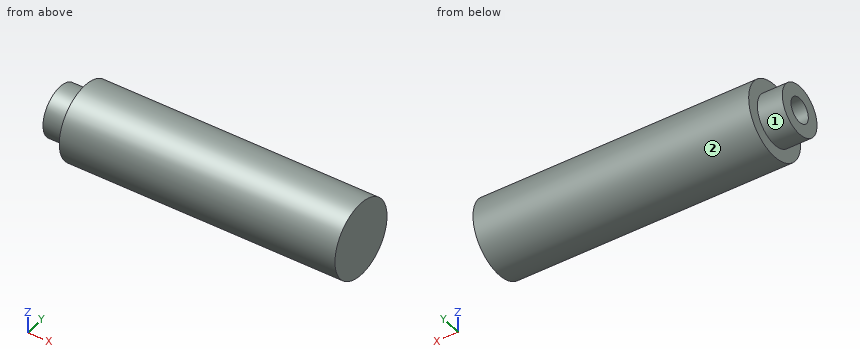
from build123d import *


with BuildPart() as part:
    # Esboço1 → Revolução1 (revolve)
    with BuildSketch(Plane.XY, mode=Mode.PRIVATE) as revolu_o1_sk:
        Polygon((-15.245, 0), (-15.245, 2.5), (-30.125, 2.5), (-30.125, 5), (-25.125, 5), (-25.125, 7.5), (30.125, 7.5), (30.125, 0), align=None)
    revolve(revolu_o1_sk.sketch.rotate(Axis((0, 0, 0), (1, 0, 0)), 90), axis=Axis((0, 0, 0), (1, 0, 0)))


solid = part.part
Could you check a few things on this model? Use its own coordinates, in mm. Face numbers are marked on the shaded views. A direction names the side the tool comes from. Coordinates: 2 decimals unless noted, no trailing zeros. Loops run counter-clockwise (first coordinate to the right, second up) from the corner with the lowest first, then second, coordinate; pieces in that order, holes last. Notation, with made-up numbers: (32.5, 12.25) -> (78.5, 12.25) arc R15 cw to (78.5, 23.25) -> close; hole circle Ø9 at (65.5, 67.5). An arc over 180 degrees is marked (long way). Answer in a Markdown table with one row per item.
(1) Imagine slicing it at A-A (y = 0). List the corners of the cut face in (x, z) for me (3 decimals), plus the area to 3 significant figures.
Results found:
| item | result |
|---|---|
| outline | (-30.125, -5) -> (-25.125, -5) -> (-25.125, -7.5) -> (30.125, -7.5) -> (30.125, 7.5) -> (-25.125, 7.5) -> (-25.125, 5) -> (-30.125, 5) -> (-30.125, 2.5) -> (-15.245, 2.5) -> (-15.245, -2.5) -> (-30.125, -2.5) -> close |
| area | 804 mm^2 |
(2) Imagine slicing it at C-C (x = -20). List the corners of the cut face in (y, z) for me, plus the area to 3 significant figures.
Results found:
| item | result |
|---|---|
| outline | circle Ø15 at (0, 0); hole circle Ø5 at (0, 0) |
| area | 157 mm^2 |
(3) If I drill on probe 1 along Z at (x, y) = (-17.5, 0.25); probe 2 along Y at (x, z) = (-18.5, 0); probe 3 along Y at (x, z) = (-26.25, 0), over which ranges is the centre line in solid material (lowest first)?
Results found:
| item | result |
|---|---|
| probe 1 | z = -7.5 to -2.49, 2.49 to 7.5 |
| probe 2 | y = -7.5 to -2.5, 2.5 to 7.5 |
| probe 3 | y = -5 to -2.5, 2.5 to 5 |
(4) Imagine slicing it at D-D (x = -11). List the corners of the cut face in (y, z) for me.
Results found:
| item | result |
|---|---|
| outline | circle Ø15 at (0, 0) |
(5) For the marked faces 1 and 2, which set-ups out of +Z, -Z, +X, -X, +Y, -Y let a thin tool reach every point of the face, with its end or its side?
Results found:
| item | result |
|---|---|
| face 1 | -X |
| face 2 | +X, -X |
(6) Will these pins go through, and if not, where does the flat tip stop? pin 1 Ø3 at (x, z) = (-18.5, -3.5) entering from +Y; pin 2 Ø2.5 at (y, z) = (0, 0.5) entering from -X (3 decimals).
Results found:
| item | result |
|---|---|
| pin 1 | stops at y = 7.23 |
| pin 2 | stops at x = -15.245 |
